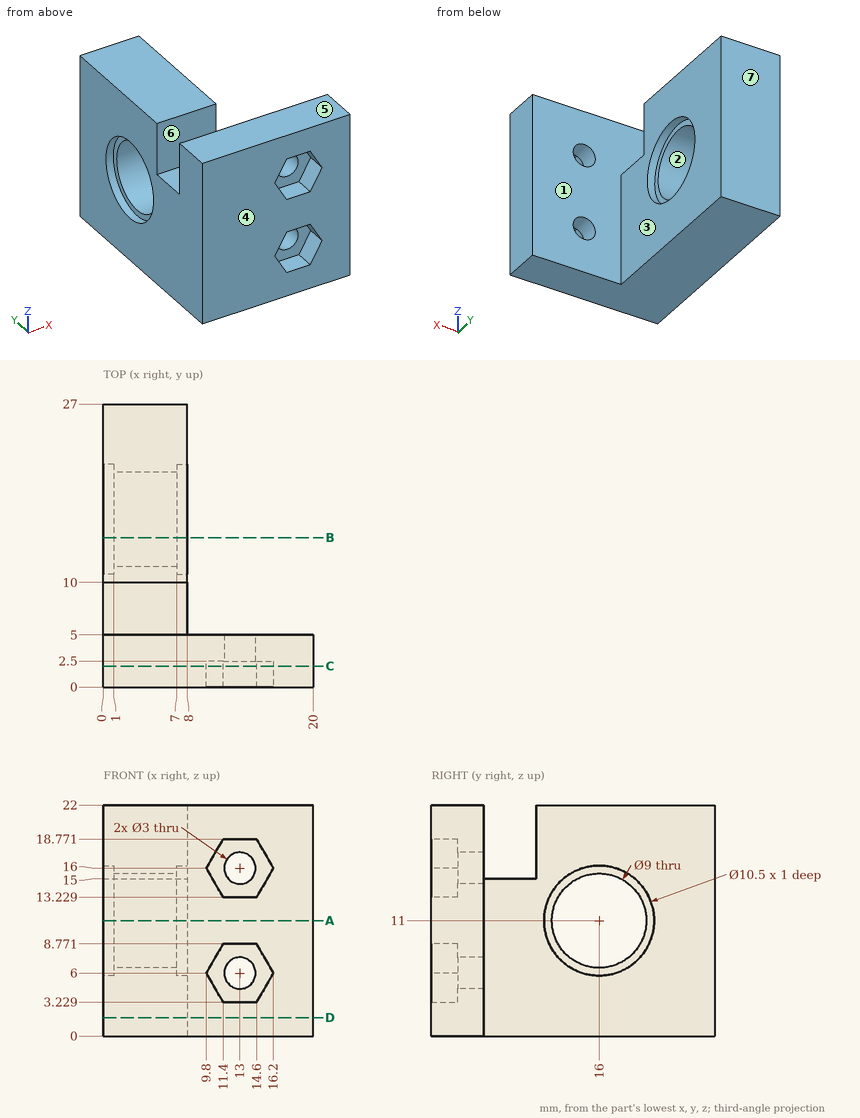
Print and shaded views of the part. All mm, measured from the part's lowest x, y and z. A direction names the side the tool comes from. Coordinates: 2 decimals unless noted, no trailing zeros. Loops run counter-clockwise (first coordinate to the right, second up) from the corner with the lowest first, then second, coordinate; pieces in that order, holes last. Notation, with made-up numbers: (70, 33.5) -> (87, 33.5) arc R24 cw to (87, 70.5) -> close; hole circle Ø4 at (-11, 12). An arc over 180 degrees is marked (long way). Use a Markdown table: item, result. Add a question column.
Item 1: Probe probe 1 along Z at (x, y) = (13, 3.35); probe 2 along Z at (x, y) = (4.75, 7.75); probe 3 along Y at (x, z) = (7.4, 11). List the from-to ranges inside material, lowest first.
Item 2: Band-saw the part on D-D on z = 1.75. Write the cut outline in (x, y), plus the area to 3 significant figures.
Item 3: Flat gauge pins, fed straight in: P1, Ø1.7, axis at x = 14, z = 5.5, coming from the -Y side; P2, Ø0.8, axis at x = 12.5, y = 1.5, coming from the -Z side; P3, Ø5, axis at x = 13, z = 6, coming from the +Y side; P4, Ø1, axis at x = 7.5, y = 8.5, coming from the +Z side. Where does each tip first touch, or does it go through?
Item 4: Which spindle directions (+Z, -Z, +X, -X, +Y, -Y) get a long thin tool onto all of the face, cutting with end or side? Do the marked faces 1, 2 and 3. Say none if no direction does.
Item 5: Band-saw the part on B-B on y = 14.25. Write the cut outline in (x, z), plus the area to 3 significant figures.
Item 6: Band-saw the part on A-A on z = 11. Write the cut outline in (x, y).
Item 7: Pull direction Y, two halves, no side cores. Call the marked faces 4, 5, 6 and 7: +Y half, -Y half, draft (parallel to the pull), parting line (faces both ways), or undercut.
Item 8: Band-saw the part on C-C on y = 2. Write the cut outline in (x, z), plus the area to 3 significant figures.
Geometry says:
| question | item | result |
|---|---|---|
| 1 | probe 1 | 0 to 4.5, 7.5 to 14.5, 17.5 to 22 |
| 1 | probe 2 | 0 to 15 |
| 1 | probe 3 | 0 to 10.75, 21.25 to 27 |
| 2 | outline | (0, 0) -> (20, 0) -> (20, 5) -> (8, 5) -> (8, 27) -> (0, 27) -> close |
| 2 | area | 276 mm² |
| 3 | P1 | y = 2.5 |
| 3 | P2 | z = 0 |
| 3 | P3 | y = 5 |
| 3 | P4 | z = 15 |
| 4 | face 1 | +Z, +X |
| 4 | face 2 | +X, -X |
| 4 | face 3 | +Z, -Z, +X, +Y |
| 5 | outline | (0, 0) -> (8, 0) -> (8, 6.05) -> (7, 6.05) -> (7, 6.85) -> (1, 6.85) -> (1, 6.05) -> (0, 6.05) -> close; (0, 15.95) -> (1, 15.95) -> (1, 15.15) -> (7, 15.15) -> (7, 15.95) -> (8, 15.95) -> (8, 22) -> (0, 22) -> close |
| 5 | area | 106 mm² |
| 6 | outline | (0, 0) -> (20, 0) -> (20, 5) -> (8, 5) -> (8, 10.75) -> (7, 10.75) -> (7, 11.5) -> (1, 11.5) -> (1, 10.75) -> (0, 10.75) -> close; (0, 21.25) -> (1, 21.25) -> (1, 20.5) -> (7, 20.5) -> (7, 21.25) -> (8, 21.25) -> (8, 27) -> (0, 27) -> close |
| 7 | face 4 | -Y half |
| 7 | face 5 | draft |
| 7 | face 6 | undercut |
| 7 | face 7 | +Y half |
| 8 | outline | (0, 0) -> (20, 0) -> (20, 22) -> (0, 22) -> close; hole (9.8, 6) -> (11.4, 3.23) -> (14.6, 3.23) -> (16.2, 6) -> (14.6, 8.77) -> (11.4, 8.77) -> close; hole (9.8, 16) -> (11.4, 13.23) -> (14.6, 13.23) -> (16.2, 16) -> (14.6, 18.77) -> (11.4, 18.77) -> close |
| 8 | area | 387 mm² |
